```python
from build123d import *
from OCP.BRepFilletAPI import BRepFilletAPI_MakeChamfer

# Parameters (mm, degrees)
ESQUISSE1_W                    = 115
ESQUISSE1_H                    = 135
BOSS_EXTRU_1_DEPTH             = 3
BOSS_EXTRU_2_DEPTH             = 10
BOSS_EXTRU_3_DEPTH             = 7
ESQUISSE5_W                    = 15
ESQUISSE5_H                    = 3
BOSS_EXTRU_4_DEPTH             = 7
CHANFREIN1_SIZE                = 5.773502692
CHANFREIN1_SIZE_2              = 10
CONG_1_R                       = 3
CHANFREIN1_OF_SYM_TRIE1_SIZE   = 5.773502692
CHANFREIN1_OF_SYM_TRIE1_SIZE_2 = 10
CONG_1_OF_SYM_TRIE1_R          = 3
CONG_2_R                       = 5


with BuildPart() as part:
    # Esquisse1 → Boss.-Extru.1 (new body)
    with BuildSketch(Plane(origin=(0, 0, 0), x_dir=(1, 0, 0), z_dir=(0, 1, 0))):
        Rectangle(ESQUISSE1_W, ESQUISSE1_H)
    extrude(amount=BOSS_EXTRU_1_DEPTH)

    # Esquisse2 → Boss.-Extru.2 (add)
    with BuildSketch(Plane(origin=(0, 3, 0), x_dir=(1, 0, 0), z_dir=(0, 1, 0))):
        Polygon((-57.5, 24.25), (-51, 24.25), (-51, 31.75), (-49, 31.75), (-49, 24.25), (-42.5, 24.25), (-42.5, 22.25), (-57.5, 22.25), align=None)
        Polygon((-42.5, 18.75), (-42.5, 20.75), (-57.5, 20.75), (-57.5, 18.75), (-51, 18.75), (-51, 11.25), (-49, 11.25), (-49, 18.75), align=None)
        Polygon((-51, -22.75), (-51, -15.25), (-49, -15.25), (-49, -22.75), (-42.5, -22.75), (-42.5, -24.75), (-57.5, -24.75), (-57.5, -22.75), align=None)
        Polygon((-57.5, -29.75), (-51, -29.75), (-51, -37.25), (-49, -37.25), (-49, -29.75), (-42.5, -29.75), (-42.5, -27.75), (-57.5, -27.75), align=None)
    boss_extru_2 = extrude(amount=BOSS_EXTRU_2_DEPTH)

    # Esquisse4 → Boss.-Extru.3 (add)
    with BuildSketch(Plane(origin=(0, 13, 0), x_dir=(1, 0, 0), z_dir=(0, 1, 0))):
        Polygon((-57.5, -27.75), (-57.5, -29.75), (-51, -29.75), (-51, -37.25), (-49, -37.25), (-49, -29.75), (-42.5, -29.75), (-42.5, -27.75), align=None)
        Polygon((-51, -22.75), (-57.5, -22.75), (-57.5, -24.75), (-42.5, -24.75), (-42.5, -22.75), (-49, -22.75), (-49, -15.25), (-51, -15.25), align=None)
    boss_extru_3 = extrude(amount=BOSS_EXTRU_3_DEPTH)

    # Esquisse5 → Boss.-Extru.4 (add)
    with BuildSketch(Plane(origin=(0, 3, 0), x_dir=(1, 0, 0), z_dir=(0, 1, 0))):
        with Locations((-50, -26.25)):
            Rectangle(ESQUISSE5_W, ESQUISSE5_H)
    boss_extru_4 = extrude(amount=BOSS_EXTRU_4_DEPTH)

    # Chanfrein1
    chanfrein1_edges_1 = [part.edges().sort_by_distance(p)[0] for p in [
        (-50, 13, -31.75),
    ]]
    chanfrein1_side_1 = [part.faces().sort_by_distance(p)[0] for p in [
        (-50, 13, -31.634529946),
    ]]
    chanfrein1_edges_2 = [part.edges().sort_by_distance(p)[0] for p in [
        (-50, 13, -11.25),
    ]]
    chanfrein1_side_2 = [part.faces().sort_by_distance(p)[0] for p in [
        (-50, 13, -11.365470054),
    ]]
    chanfrein1_edges_3 = [part.edges().sort_by_distance(p)[0] for p in [
        (-50, 20, 37.25),
    ]]
    chanfrein1_side_3 = [part.faces().sort_by_distance(p)[0] for p in [
        (-50, 20, 37.134529946),
    ]]
    chanfrein1_edges_4 = [part.edges().sort_by_distance(p)[0] for p in [
        (-50, 20, 15.25),
    ]]
    chanfrein1_side_4 = [part.faces().sort_by_distance(p)[0] for p in [
        (-50, 20, 15.365470054),
    ]]
    chanfrein1 = BRepFilletAPI_MakeChamfer(part.part.solid().wrapped)
    for e in chanfrein1_edges_1:
        chanfrein1.Add(CHANFREIN1_SIZE - 0.0001, CHANFREIN1_SIZE_2 - 0.0001, e.wrapped, chanfrein1_side_1[0].wrapped)
    for e in chanfrein1_edges_2:
        chanfrein1.Add(CHANFREIN1_SIZE - 0.0001, CHANFREIN1_SIZE_2 - 0.0001, e.wrapped, chanfrein1_side_2[0].wrapped)
    for e in chanfrein1_edges_3:
        chanfrein1.Add(CHANFREIN1_SIZE - 0.0001, CHANFREIN1_SIZE_2 - 0.0001, e.wrapped, chanfrein1_side_3[0].wrapped)
    for e in chanfrein1_edges_4:
        chanfrein1.Add(CHANFREIN1_SIZE - 0.0001, CHANFREIN1_SIZE_2 - 0.0001, e.wrapped, chanfrein1_side_4[0].wrapped)
    add(Compound.cast(chanfrein1.Shape()), mode=Mode.REPLACE)  # a hair under: the kernel refuses the full size

    # Congé1
    cong_1_edges = [part.edges().sort_by_distance(p)[0] for p in [
        (-57.5, 20, 28.75),
        (-42.5, 20, 28.75),
        (-57.5, 20, 23.75),
        (-42.5, 20, 23.75),
        (-57.5, 13, -23.25),
        (-42.5, 13, -23.25),
        (-42.5, 13, -19.75),
        (-57.5, 13, -19.75),
    ]]
    fillet(cong_1_edges, radius=CONG_1_R)

    # Symétrie1: Boss.-Extru.2, Boss.-Extru.3, Boss.-Extru.4 across plane
    add(boss_extru_2.mirror(Plane(origin=(0, 0, 0), x_dir=(0, 0, 1), z_dir=(1, 0, 0))))
    add(boss_extru_3.mirror(Plane(origin=(0, 0, 0), x_dir=(0, 0, 1), z_dir=(1, 0, 0))))
    add(boss_extru_4.mirror(Plane(origin=(0, 0, 0), x_dir=(0, 0, 1), z_dir=(1, 0, 0))))

    # Chanfrein1 of Symétrie1
    chanfrein1_of_sym_trie1_edges_1 = [part.edges().sort_by_distance(p)[0] for p in [
        (50, 13, -31.75),
    ]]
    chanfrein1_of_sym_trie1_side_1 = [part.faces().sort_by_distance(p)[0] for p in [
        (50, 13, -31.634529946),
    ]]
    chanfrein1_of_sym_trie1_edges_2 = [part.edges().sort_by_distance(p)[0] for p in [
        (50, 13, -11.25),
    ]]
    chanfrein1_of_sym_trie1_side_2 = [part.faces().sort_by_distance(p)[0] for p in [
        (50, 13, -11.365470054),
    ]]
    chanfrein1_of_sym_trie1_edges_3 = [part.edges().sort_by_distance(p)[0] for p in [
        (50, 20, 37.25),
    ]]
    chanfrein1_of_sym_trie1_side_3 = [part.faces().sort_by_distance(p)[0] for p in [
        (50, 20, 37.134529946),
    ]]
    chanfrein1_of_sym_trie1_edges_4 = [part.edges().sort_by_distance(p)[0] for p in [
        (50, 20, 15.25),
    ]]
    chanfrein1_of_sym_trie1_side_4 = [part.faces().sort_by_distance(p)[0] for p in [
        (50, 20, 15.365470054),
    ]]
    chanfrein1_of_sym_trie1 = BRepFilletAPI_MakeChamfer(part.part.solid().wrapped)
    for e in chanfrein1_of_sym_trie1_edges_1:
        chanfrein1_of_sym_trie1.Add(CHANFREIN1_OF_SYM_TRIE1_SIZE - 0.0001, CHANFREIN1_OF_SYM_TRIE1_SIZE_2 - 0.0001, e.wrapped, chanfrein1_of_sym_trie1_side_1[0].wrapped)
    for e in chanfrein1_of_sym_trie1_edges_2:
        chanfrein1_of_sym_trie1.Add(CHANFREIN1_OF_SYM_TRIE1_SIZE - 0.0001, CHANFREIN1_OF_SYM_TRIE1_SIZE_2 - 0.0001, e.wrapped, chanfrein1_of_sym_trie1_side_2[0].wrapped)
    for e in chanfrein1_of_sym_trie1_edges_3:
        chanfrein1_of_sym_trie1.Add(CHANFREIN1_OF_SYM_TRIE1_SIZE - 0.0001, CHANFREIN1_OF_SYM_TRIE1_SIZE_2 - 0.0001, e.wrapped, chanfrein1_of_sym_trie1_side_3[0].wrapped)
    for e in chanfrein1_of_sym_trie1_edges_4:
        chanfrein1_of_sym_trie1.Add(CHANFREIN1_OF_SYM_TRIE1_SIZE - 0.0001, CHANFREIN1_OF_SYM_TRIE1_SIZE_2 - 0.0001, e.wrapped, chanfrein1_of_sym_trie1_side_4[0].wrapped)
    add(Compound.cast(chanfrein1_of_sym_trie1.Shape()), mode=Mode.REPLACE)  # a hair under: the kernel refuses the full size

    # Congé1 of Symétrie1
    cong_1_of_sym_trie1_edges = [part.edges().sort_by_distance(p)[0] for p in [
        (57.5, 20, 28.75),
        (42.5, 20, 28.75),
        (57.5, 20, 23.75),
        (42.5, 20, 23.75),
        (57.5, 13, -23.25),
        (42.5, 13, -23.25),
        (42.5, 13, -19.75),
        (57.5, 13, -19.75),
    ]]
    fillet(cong_1_of_sym_trie1_edges, radius=CONG_1_OF_SYM_TRIE1_R)

    # Congé2
    cong_2_edges = [part.edges().sort_by_distance(p)[0] for p in [
        (57.5, 1.5, 67.5),
        (-57.5, 1.5, 67.5),
        (-57.5, 1.5, -67.5),
        (57.5, 1.5, -67.5),
    ]]
    fillet(cong_2_edges, radius=CONG_2_R)


solid = part.part
```
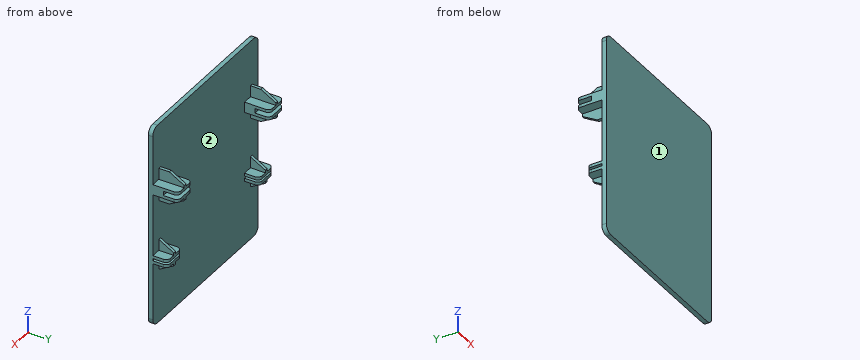
Read the model definition and answer for the solid it produces. Units are mm, in the model's axes. Face numbers are marked on the shaded views. Round coordinates to 2 decimals unless told otherwise and drop trailing zeros. Write each loop counter-clockwise with the first axis right and the second up, starting at its lowest first coordinate (ties: lowest second). Pieces come first, ordered by that corner, then holes. Notation, with made-up numbers: M 71,-30 L 76,-30 A27 ccw 76,8 Z; hole C -4,-34.75 d1. An arc over 180 degrees is marked long. One line per item, written item: value.
Q1. Find section C-C on z = -55. Write down the section's boundary in (x, y).
Data:
outline: M -57.5,0 L 57.5,0 L 57.5,3 L -57.5,3 Z
Q2. Find section B-B on x = 28.5. Write down the section's boundary in (y, z), plus the area to 3 significant figures.
Data:
outline: M 0,-67.5 L 3,-67.5 L 3,67.5 L 0,67.5 Z
area: 405 mm2
Q3. For a pull along X with two mould halves and no side action, classify the marked faces 1 and 2 as +X half, -X half, draft (parallel to the pull), parting line (faces both ways), or undercut.
Data:
face 1: draft
face 2: undercut
Q4. Straight lines are drawn through the part: line 1 (Z direction, x = 46.5, y = 10.25); line 2 (X direction, y = 8.5, z = 16); line 3 (X direction, y = 12.75, z = 24). For each, find the intervals that lie inside material, in ascending order. Write a range as [from, to].
Data:
line 1: [-24.25, -22.25], [-20.75, -18.75], [22.75, 24.75], [27.75, 29.75]
line 2: [-51, -49], [49, 51]
line 3: [-57.5, -42.5], [42.5, 57.5]
Q5. Find section A-A on y = 7.25. Count the separate pieces of the cut face and the enclosed holes in it, plus the area to 3 significant figures.
Data:
separate pieces: 6
enclosed holes: 0
area: 430 mm2
Q6. Flat-ended cylindrical pins translate along their axes: pin 1 Ø7 at (x, y) = (-47, 9.5) entering from -Z; pin 2 Ø8 at (x, y) = (50.5, 15.5) entering from -Z; pin 3 Ø8 at (x, y) = (-48, 14) entering from -Z; pin 4 Ø10 at (x, y) = (20.5, 9) entering from +Z. Find the tip coordinate at first contact, or state that the pin passes through.
Data:
pin 1: z = -29.66
pin 2: z = -26.84
pin 3: z = -27.64
pin 4: through
